Answer from the drawing. Dimensions are ordinates in mm from the lowest x, y and z of the part. Coordinates: 2 decimals unless noted, no trailing zeros. Order: outer loops, then holes, each group sorted by start corner. A loop starts at its lowest first (then second) coordinate and runs counter-clockwise, first axis right, second up.
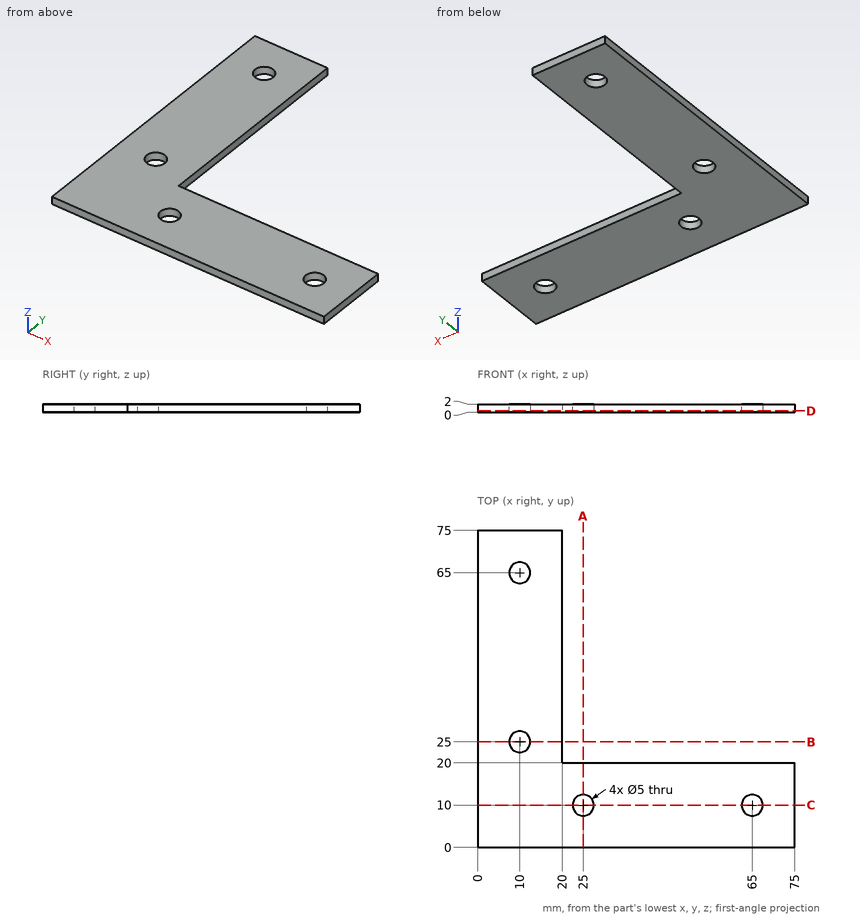
1. The part is cut by section C-C (y = 10). Determine the outline of the cut face in (x, z).
2. Consider probe 1 along Y at (x, z) = (10, 0.5); probe 2 along Y at (x, z) = (65, 0.75); probe 3 along Y at (x, z) = (9, 0.25). Determine where each line is inside the solid, lowest interval first.
3. The part is cut by section A-A (x = 25). Determine the outline of the cut face in (y, z).
4. The part is cut by section D-D (z = 0.4). Determine the outline of the cut face in (x, y).
5. A flat-ended cylindrical pin translates along its axis: pin 1 (3 mm diameter, centred on x = 10, y = 65, fed in from +Z). Find the tip coordinate at first contact, or state that the pin passes through.
Worked out:
1. outline: (0, 0) - (22.5, 0) - (22.5, 2) - (0, 2) - close; (27.5, 0) - (62.5, 0) - (62.5, 2) - (27.5, 2) - close; (67.5, 0) - (75, 0) - (75, 2) - (67.5, 2) - close
2. probe 1: y = 0 to 22.5, 27.5 to 62.5, 67.5 to 75
2. probe 2: y = 0 to 7.5, 12.5 to 20
2. probe 3: y = 0 to 22.71, 27.29 to 62.71, 67.29 to 75
3. outline: (0, 0) - (7.5, 0) - (7.5, 2) - (0, 2) - close; (12.5, 0) - (20, 0) - (20, 2) - (12.5, 2) - close
4. outline: (0, 0) - (75, 0) - (75, 20) - (20, 20) - (20, 75) - (0, 75) - close; hole circle Ø5 at (10, 25); hole circle Ø5 at (10, 65); hole circle Ø5 at (25, 10); hole circle Ø5 at (65, 10)
5. pin 1: passes through
